Here's how the part is built. I have some questions about the finished solid (model axes, mm). A direction names the side the tool comes from. Give positions to 0.01 mm unless a question says otherwise; leave off trailing zeros. Loops run counter-clockwise (first coordinate to the right, second up) from the corner with the lowest first, then second, coordinate; pieces in that order, holes last. Notation, with made-up numbers: (54, -10.75) - (74, -10.75) arc R28 ccw to (74, 16.25) - close; hole circle Ø4 at (60, 39.25). An arc over 180 degrees is marked (long way). Return JSON: item names as keys, results as strings. Group by question number.
(1) I need wall thicknesses on probe 1 along Z at (x, y) = (34, 10); probe 2 along Z at (x, y) = (-3.5, -25.5); probe 3 along X at (y, z) = (-0.5, 2). Which ranges of each line are inside material? Lowest first, please. Write a range as [from, to].
(2) On a 3-axis mill with a long thin cutter (end or side, diameter ignored), from which of +Z, -Z, +X, -X, +Y, -Y can I reach the whole of each face in a straight line? I mean faces 1 (the cylindrical face through (-39.3, -2.89, 12.32)), 2 (the flat face through (7.195, 2, 30)), 3 (the flat face through (24, 16.607, 30)), 4 (the flat face through (24, -11.58, 30)), 5 (the flat face through (42.084, 2, 30)). Say none if no direction works.
(3) If we mould it in two halves opening along Z, with no side actions, what happens to faces 6 (the flat face through (66.138, -1, 12)), 7 (the cylindrical face through (39.39, -0.65, 11.15)), 8 (the flat face through (24, 3, 35)), 9 (the flat face through (-1, 1, 0))? For each: released by +Z, released by -Z, zero draft, split by the parting line, or undercut.
(4) If we section it at A-A (y = 2.5): Please give me the cut outline in (x, z), then the cut area to 3 significant figures.
(5) If we section it at C-C (x = -22.5): Please give me the cut outline in (y, z), then the cut area to 3 significant figures.
(6) For P1, Ø3, axis at y = -1.5, z = 30.5, coming from the +X side; P2, Ø23, axis at x = -30.06, y = 0.94, coming from the +Z side; P3, Ø8, axis at x = 29, z = 32, coming from the +Y side; P4, Ø4, axis at y = -20, z = 26, coming from the +X side, each with a flat end and sliding along its axis, tell me the tip position at first contact or that it passes through.
(7) If we section it at D-D (y = 24): Please give me the cut outline in (x, z), then the cut area to 3 significant figures.
(8) If we section it at B-B (x = 9.5): Please give me the cut outline in (y, z), then the cut area to 3 significant figures.
```python
from build123d import *

# Parameters (mm, degrees)
SKETCH1_W              = 132.276038998
SKETCH1_H              = 92.368395504
BOSS_EXTRUDE1_DEPTH    = 25
F_20_0MM_DOWEL_HOLE1_D = 20
F_10_0MM_DOWEL_HOLE1_D = 10
SKETCH8_W              = 34.889280452
SKETCH8_H              = 28.187384772
BOSS_EXTRUDE2_DEPTH    = 10


with BuildPart() as part:
    # Sketch1 → Boss-Extrude1 (new body)
    with BuildSketch(Plane.XY):
        Rectangle(SKETCH1_W, SKETCH1_H)
    extrude(amount=BOSS_EXTRUDE1_DEPTH)

    # Ø20.0mm Dowel Hole1 (through all)
    with Locations(Plane.XY.offset(25)):
        with Locations((-30.059973271, 0.936294249)):
            Hole(F_20_0MM_DOWEL_HOLE1_D / 2)

    # Ø10.0mm Dowel Hole1 (through all)
    with Locations(Plane(origin=(0, 46.184197752, 0), x_dir=(1, 0, 0), z_dir=(0, 1, 0))):
        with Locations((34.396494005, -11.366591172)):
            Hole(F_10_0MM_DOWEL_HOLE1_D / 2)

    # Sketch8 → Boss-Extrude2 (add)
    with BuildSketch(Plane.XY.offset(25)):
        with Locations((24.639322353, 2.51321088)):
            Rectangle(SKETCH8_W, SKETCH8_H)
    extrude(amount=BOSS_EXTRUDE2_DEPTH)


solid = part.part
```
Values:
{
 "1": {"probe 1": "[0, 6.38], [16.35, 35]", "probe 2": "[0, 25]", "probe 3": "[-66.14, -39.96], [-20.16, 66.14]"},
 "2": {"face 1": "+Z, -Z", "face 2": "+Z, -X, +Y, -Y", "face 3": "+Z, +X, -X, +Y", "face 4": "+Z, +X, -X, -Y", "face 5": "+Z, +X, +Y, -Y"},
 "3": {"face 6": "zero draft", "face 7": "undercut", "face 8": "released by +Z", "face 9": "released by -Z"},
 "4": {"outline": "(-66.14, 0) - (-39.94, 0) - (-39.94, 25) - (-66.14, 25) - close; (-20.18, 0) - (66.14, 0) - (66.14, 25) - (42.08, 25) - (42.08, 35) - (7.19, 35) - (7.19, 25) - (-20.18, 25) - close; hole circle Ø10 at (34.4, 11.37)", "area": "3,080 mm2"},
 "5": {"outline": "(-46.18, 0) - (-5.61, 0) - (-5.61, 25) - (-46.18, 25) - close; (7.48, 0) - (46.18, 0) - (46.18, 25) - (7.48, 25) - close", "area": "1,980 mm2"},
 "6": {"P1": "x = 42.08", "P2": "z = 25", "P3": "y = 16.61", "P4": "x = 66.14"},
 "7": {"outline": "(-66.14, 0) - (66.14, 0) - (66.14, 25) - (-66.14, 25) - close; hole circle Ø10 at (34.4, 11.37)", "area": "3,230 mm2"},
 "8": {"outline": "(-46.18, 0) - (46.18, 0) - (46.18, 25) - (16.61, 25) - (16.61, 35) - (-11.58, 35) - (-11.58, 25) - (-46.18, 25) - close", "area": "2,590 mm2"}
}
